```python
from build123d import *

# Parameters (mm, degrees)
F1_W     = 3.175
F1_H     = 9.525
F2_DEPTH = 6.35
F3_R     = 1.5875
F4_DEPTH = 9.525


with BuildPart() as f2:
    # F1 (on Top) → F2 (new body)
    with BuildSketch(Plane.XY):
        with Locations((-11.1125, 1.5875)):
            Rectangle(F1_W, F1_H)
        with Locations((-7.9375, 1.5875)):
            Rectangle(F1_W, F1_H)
        with BuildLine():
            ThreePointArc((-3.175, 0), (0, 3.175), (3.175, 0))
            Line((3.175, 0), (3.175, -3.175))
            Line((3.175, -3.175), (6.35, -3.175))
            Line((6.35, -3.175), (6.35, 0))
            ThreePointArc((6.35, 0), (4.4901280605, 4.4901280605), (0, 6.35))
            Line((0, 6.35), (-6.35, 6.35))
            Line((-6.35, 6.35), (-6.35, -3.175))
            Line((-6.35, -3.175), (-3.175, -3.175))
            Line((-3.175, -3.175), (-3.175, 0))
        make_face()
    extrude(amount=F2_DEPTH)

    # F3 (on face) → F4 (cut, through all)
    with BuildSketch(Plane.XZ.offset(3.175)):
        with Locations((-7.9375, 3.175)):
            Circle(F3_R)
    extrude(amount=-F4_DEPTH, mode=Mode.SUBTRACT)


solid = f2.part
```
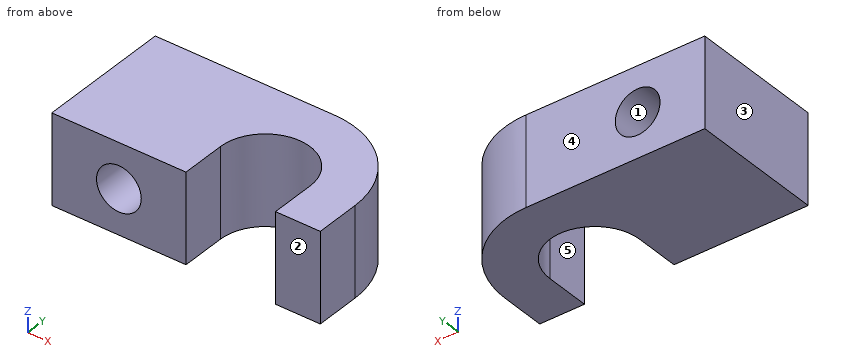
Can you work these out from the model? Positions are in its coordinate system, mm. Face numbers are marked on the shaded views. A direction names the side the tool comes from. Coordinates: 2 decimals unless noted, no trailing zeros. Loops run counter-clockwise (first coordinate to the right, second up) from the corner with the lowest first, then second, coordinate; pieces in that order, holes last.
1) Imagine slicing it at B-B on z = 4.5. List the corners of the cut face in (x, y) for me (3 decimals).
2) Imagine slicing it at A-A on y = -0.5. State how many separate pieces and enclosed holes the cut face has, plus the area to 3 significant figures.
3) Thinking about a two-plate mould opening in X: for the marked faces 1, 2 and 3, which applies, pulls with the +X half, pulls with the -X half, needs draft (parallel to the pull), parting line crosses it, or undercut?
4) I need wall thicknesses on probe 1 along X at (y, z) = (-1, 3) (3 decimals); probe 2 along X at (y, z) = (-2.5, 4.25) (3 decimals); probe 3 along X at (y, z) = (1, 5). Which ranges of each line are inside material? Lowest first, please.
5) Which directions (+Z, -Z, +X, -X, +Y, -Y) give clear straight access to the entire face, cutting with the end or side of a thin tool? Please do the marked faces 4 and 5.
6) Imagine slicing it at C-C on x = -1. List the corners of the cut face in (y, z) for me.
7) Imagine slicing it at D-D on z = 3.5. List the corners of the cut face in (x, y) for me (3 decimals).
Completed:
1. outline: (-12.7, -3.175) - (-8.812, -3.175) - (-8.812, 6.35) - (-12.7, 6.35) - close; (-7.063, -3.175) - (-3.175, -3.175) - (-3.175, 0) arc R3.175 cw to (3.175, 0) - (3.175, -3.175) - (6.35, -3.175) - (6.35, 0) arc R6.35 ccw to (0, 6.35) - (-7.063, 6.35) - close
2. separate pieces: 2
2. enclosed holes: 1
2. area: 72.7 mm2
3. face 1: undercut
3. face 2: needs draft
3. face 3: pulls with the -X half
4. probe 1: x = -12.7 to -9.515, -6.36 to -3.175, 3.175 to 6.35
4. probe 2: x = -12.7 to -9.106, -6.769 to -3.175, 3.175 to 6.35
4. probe 3: x = -12.7 to -3.01, 3.01 to 6.27
5. face 4: +Z, -Z, +X, -X, +Y
5. face 5: +Z, -Z, -Y
6. outline: (3.01, 0) - (6.35, 0) - (6.35, 6.35) - (3.01, 6.35) - close
7. outline: (-12.7, -3.175) - (-9.491, -3.175) - (-9.491, 6.35) - (-12.7, 6.35) - close; (-6.384, -3.175) - (-3.175, -3.175) - (-3.175, 0) arc R3.175 cw to (3.175, 0) - (3.175, -3.175) - (6.35, -3.175) - (6.35, 0) arc R6.35 ccw to (0, 6.35) - (-6.384, 6.35) - close
